Work out the finished part from the listing and answer in its coordinate system (mm). Round coordinates to 2 decimals unless told otherwise and drop trailing zeros. Loops run counter-clockwise (first coordinate to the right, second up) from the corner with the lowest first, then second, coordinate; pieces in that order, holes last.
```python
from build123d import *

# Parameters (mm, degrees)
BOSS_EXTRUDE1_DEPTH             = 47.625
SKETCH2_R                       = 1.75
CUT_EXTRUDE1_DEPTH              = 6
CHAMFER1_SIZE                   = 2.54
CHAMFER2_SIZE                   = 2.54
SKETCH3_R                       = 3.5
SKETCH3_R_2                     = 1.75
BOSS_EXTRUDE2_DEPTH             = 7
BOSS_EXTRUDE2_DIRECTION_2_REACH = 50.212
CHAMFER3_SIZE                   = 1


with BuildPart() as part:
    # Sketch1 → Boss-Extrude1 (new, symmetric)
    with BuildSketch(Plane(origin=(0, 0, 0), x_dir=(0, 0, -1), z_dir=(1, 0, 0))):
        Polygon((-2, -3), (-4.5, 0), (-2, 3), (2, 3), (4.5, 0), (2, -3), align=None)
    extrude(amount=BOSS_EXTRUDE1_DEPTH, both=True)

    # Sketch2 → Cut-Extrude1 (cut)
    with BuildSketch(Plane.XZ.offset(3)):
        with Locations(Location((42.875, 0, 0), (0, 0, 270))):
            Circle(SKETCH2_R)
    cut_extrude1 = extrude(amount=-CUT_EXTRUDE1_DEPTH, mode=Mode.SUBTRACT)

    # Chamfer1
    chamfer1_edges = [part.edges().sort_by_distance(p)[0] for p in [
        (47.625, -1.5, -3.25),
        (47.625, -3, 0),
        (47.625, -1.5, 3.25),
        (47.625, 1.5, 3.25),
        (47.625, 3, 0),
        (47.625, 1.5, -3.25),
    ]]
    chamfer(chamfer1_edges, length=CHAMFER1_SIZE)

    # Mirror4: Cut-Extrude1 across plane
    add(cut_extrude1.mirror(Plane(origin=(0, 0, 0), x_dir=(0, 0, 1), z_dir=(1, 0, 0))), mode=Mode.SUBTRACT)

    # Chamfer2
    chamfer2_edges = [part.edges().sort_by_distance(p)[0] for p in [
        (-47.625, 1.5, 3.25),
        (-47.625, -1.5, 3.25),
        (-47.625, -3, 0),
        (-47.625, -1.5, -3.25),
        (-47.625, 1.5, -3.25),
        (-47.625, 3, 0),
    ]]
    chamfer(chamfer2_edges, length=CHAMFER2_SIZE)

    # Sketch3 → Boss-Extrude2 (add)
    with BuildSketch(Plane(origin=(0, 3, 0), x_dir=(1, 0, 0), z_dir=(0, 1, 0))):
        with Locations(Location((-42.875, 0, 0), (0, 0, 270))):
            Circle(SKETCH3_R)
        with Locations(Location((-42.875, 0, 0), (0, 0, 90))):
            Circle(SKETCH3_R_2, mode=Mode.SUBTRACT)
    extrude(amount=BOSS_EXTRUDE2_DEPTH)

    # Sketch3 → Boss-Extrude2 direction 2 (add, up to next)
    with BuildSketch(Plane(origin=(0, 3, 0), x_dir=(1, 0, 0), z_dir=(0, 1, 0)), mode=Mode.PRIVATE) as boss_extrude2_direction_2_sk1:
        with Locations(Location((-42.875, 0, 0), (0, 0, 270))):
            Circle(SKETCH3_R)
        with Locations(Location((-42.875, 0, 0), (0, 0, 90))):
            Circle(SKETCH3_R_2, mode=Mode.SUBTRACT)
    boss_extrude2_direction_2_tool1 = extrude(boss_extrude2_direction_2_sk1.sketch, amount=-BOSS_EXTRUDE2_DIRECTION_2_REACH, mode=Mode.PRIVATE) - part.part
    add(boss_extrude2_direction_2_tool1.solids().sort_by_distance((-42.875, 3, -3.401005))[0])

    # Chamfer3
    chamfer3_edges = [part.edges().sort_by_distance(p)[0] for p in [
        (-42.875, 10, -3.5),
    ]]
    chamfer(chamfer3_edges, length=CHAMFER3_SIZE)


solid = part.part
```
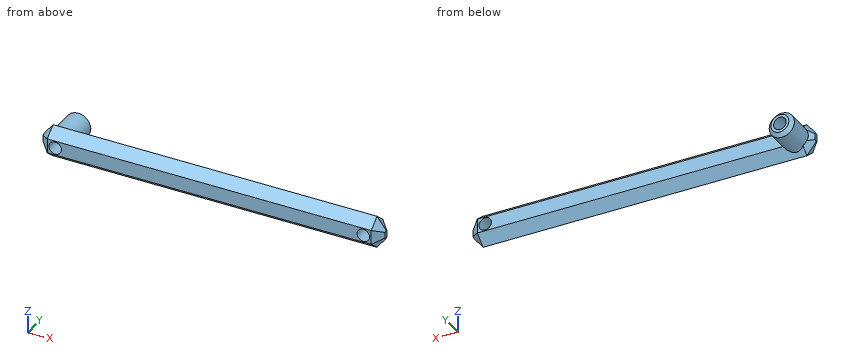
1. Find section B-B (x = -33). Write down the section's boundary in (y, z), then the cut area to 3 significant figures.
Answer key:
outline: (-3, -2) - (0, -4.5) - (3, -2) - (3, 2) - (0, 4.5) - (-3, 2) - close
area: 39.0 mm2
2. Given pin 1 (5 mm diameter, centred on x = 26.5, y = -1, fed in from +Z); pin 2 (3 mm diameter, centred on x = 9, z = -3, fed in from +Y); pin 3 (1 mm diameter, centred on y = 5, z = -3, fed in from +X); pin 4 (3 mm diameter, centred on x = -42.875, z = 0, fed in from +Y), each flat-ended and moving along its own axis, determine where each tip first touches the part or whether it passes through.
Answer key:
pin 1: stops at z = 4.5
pin 2: stops at y = 3
pin 3: stops at x = -40.43
pin 4: passes through
3. Find section A-A (z = 0). Write down the section's boundary in (x, y) (3 decimals).
Answer key:
outline: (-47.625, -0.46) - (-45.085, -3) - (-44.625, -3) - (-44.625, 10) - (-45.375, 10) - (-46.375, 9) - (-46.375, 1.71) - (-47.625, 0.46) - close; (-41.125, -3) - (41.125, -3) - (41.125, 3) - (-39.375, 3) - (-39.375, 9) - (-40.375, 10) - (-41.125, 10) - close; (44.625, -3) - (45.085, -3) - (47.625, -0.46) - (47.625, 0.46) - (45.085, 3) - (44.625, 3) - close
4. Consider probe 1 along X at (y, z) = (7, 0) (3 decimals); probe 2 along X at (y, z) = (0.5, 0) (3 decimals); probe 3 along X at (y, z) = (0, -0.5) (3 decimals). Determine where each line is inside the solid, lowest interval first.
Answer key:
probe 1: x = -46.375 to -44.625, -41.125 to -39.375
probe 2: x = -47.585 to -44.625, -41.125 to 41.125, 44.625 to 47.585
probe 3: x = -47.625 to -44.552, -41.198 to 41.198, 44.552 to 47.625
